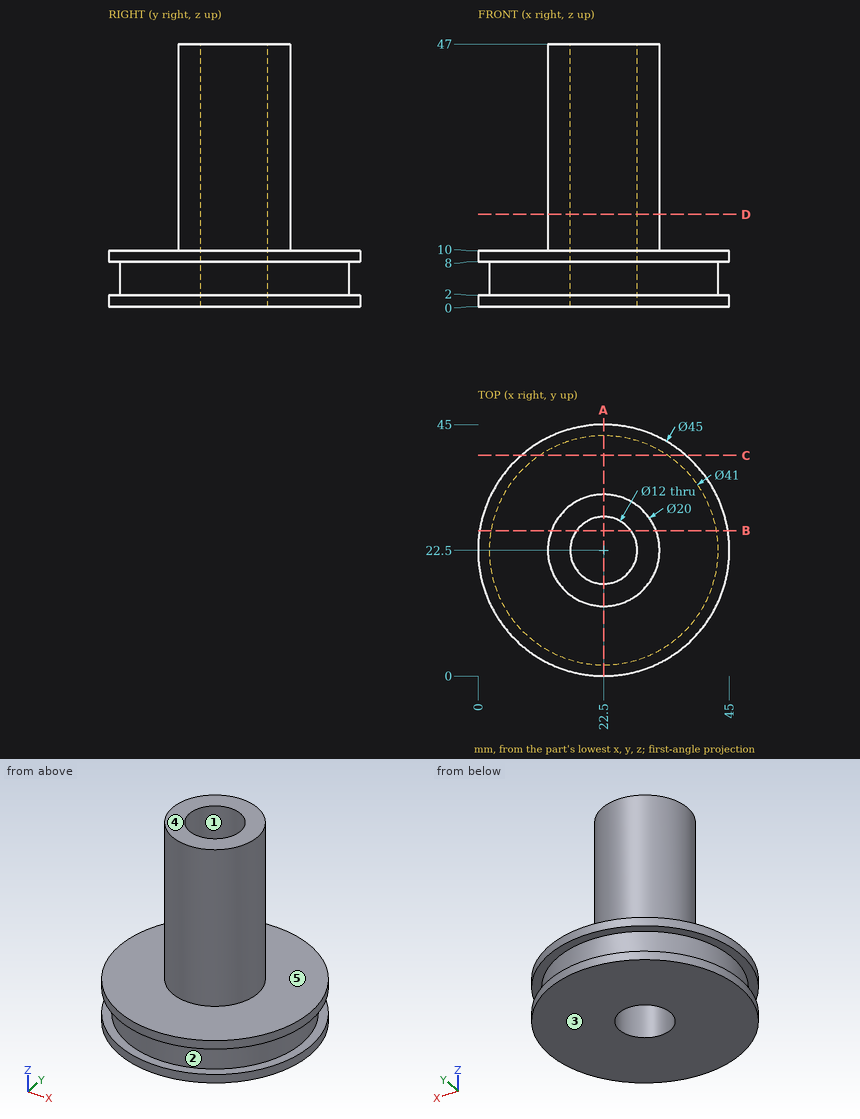
Geometry: see drawing. Coordinates: mm, zero at the bounding-box minimum. A direction names the side the tool comes from. Give positions to 0.01 mm unless a question says otherwise; leave off trailing zeros. Write each loop counter-clockwise with the first axis right and the second up, starting at its lowest first coordinate (ties: lowest second). Pieces come first, ordered by that corner, then holes. Notation, with made-up numbers: (-29.5, 77) -> (5.5, 77) arc R22 cw to (5.5, 114) -> close; hole circle Ø3 at (3.25, 50.25). An arc over 180 degrees is marked (long way). Use one line per item in the form item = value. Start each with the question number.
1) Section query D-D on z = 16.5. Return the cut outline in (x, y).
2) Section query B-B on y = 26. Return the cut outline in (x, z), then the cut area to 3 significant figures.
3) Ray query, probe 1 along Y at (x, z) = (22.5, 19.5); probe 2 along Z at (x, y) = (31, 37); probe 3 along X at (y, z) = (18, 11). Return the intervals inside material, ascending. Write a range as from..to.
4) Set-up query: the marked faces 4 and 5. Return all of +Z, -Z, +X, -X, +Y, -Y with unobstructed straight access to the full face (end or side cutting, diameter ignored); none if empty.
5) Section query A-A on x = 22.5. Return the cut outline in (y, z).
6) Pin query (flat end, axial travel): pin 1 (6 mm diameter, centred on x = 28.5, z = 20.5, fed in from +Y); pin 2 (6 mm diameter, centred on y = 5, z = 9, fed in from -X); pin 3 (8 mm diameter, centred on x = 12, z = 29.5, fed in from +Y); pin 4 (10 mm diameter, centred on y = 5, z = 20, fed in from +X). Return the tip coordinate at first contact, or that it passes through.
7) Section query C-C on y = 39.5. Return the cut outline in (x, z).
8) Draft query along X for the marked faces 1, 2 and 3. Return one class per face: pulls with the +X half, pulls with the -X half, needs draft (parallel to the pull), parting line crosses it, or undercut.
Outcome:
q1.outline = circle Ø20 at (22.5, 22.5); hole circle Ø12 at (22.5, 22.5)
q2.outline = (0.27, 0) -> (17.63, 0) -> (17.63, 47) -> (13.13, 47) -> (13.13, 10) -> (0.27, 10) -> (0.27, 8) -> (2.3, 8) -> (2.3, 2) -> (0.27, 2) -> close; (27.37, 0) -> (44.73, 0) -> (44.73, 2) -> (42.7, 2) -> (42.7, 8) -> (44.73, 8) -> (44.73, 10) -> (31.87, 10) -> (31.87, 47) -> (27.37, 47) -> close
q2.area = 655 mm^2
q3.probe_1 = 12.5..16.5, 28.5..32.5
q3.probe_2 = 0..10
q3.probe_3 = 13.57..18.53, 26.47..31.43
q4.face_4 = +Z, +X, -X, +Y, -Y
q4.face_5 = +Z
q5.outline = (0, 0) -> (16.5, 0) -> (16.5, 47) -> (12.5, 47) -> (12.5, 10) -> (0, 10) -> (0, 8) -> (2, 8) -> (2, 2) -> (0, 2) -> close; (28.5, 0) -> (45, 0) -> (45, 2) -> (43, 2) -> (43, 8) -> (45, 8) -> (45, 10) -> (32.5, 10) -> (32.5, 47) -> (28.5, 47) -> close
q6.pin_1 = 32.04
q6.pin_2 = 5.3
q6.pin_3 = 30.1
q6.pin_4 = through
q7.outline = (7.76, 0) -> (37.24, 0) -> (37.24, 2) -> (33.96, 2) -> (33.96, 8) -> (37.24, 8) -> (37.24, 10) -> (7.76, 10) -> (7.76, 8) -> (11.04, 8) -> (11.04, 2) -> (7.76, 2) -> close
q8.face_1 = undercut
q8.face_2 = parting line crosses it
q8.face_3 = needs draft
